```python
from build123d import *

# Parameters (mm, degrees)
SKETCH1_R           = 200
BOSS_EXTRUDE1_DEPTH = 5
CUT_EXTRUDE1_REACH  = 7
SKETCH2_R           = 5
CUT_EXTRUDE2_REACH  = 7
SKETCH3_R           = 2.75
CUT_EXTRUDE3_REACH  = 7
SKETCH4_R           = 2


with BuildPart() as part:
    # Sketch1 → Boss-Extrude1 (new body)
    with BuildSketch(Plane.XY):
        Circle(SKETCH1_R)
    extrude(amount=BOSS_EXTRUDE1_DEPTH)

    # Sketch2 → Cut-Extrude1 (cut, up to next)
    with BuildSketch(Plane.XY.offset(5), mode=Mode.PRIVATE) as cut_extrude1_sk1:
        with Locations((0, 180)):
            Circle(SKETCH2_R)
    cut_extrude1_tool1 = extrude(cut_extrude1_sk1.sketch, amount=-CUT_EXTRUDE1_REACH, mode=Mode.PRIVATE) & part.part
    add(cut_extrude1_tool1.solids().sort_by_distance((0, 180, 5))[0], mode=Mode.SUBTRACT)
    # Sketch2 → Cut-Extrude1 (cut, up to next)
    with BuildSketch(Plane.XY.offset(5), mode=Mode.PRIVATE) as cut_extrude1_sk2:
        with Locations((155.884572681, -90)):
            Circle(SKETCH2_R)
    cut_extrude1_tool2 = extrude(cut_extrude1_sk2.sketch, amount=-CUT_EXTRUDE1_REACH, mode=Mode.PRIVATE) & part.part
    add(cut_extrude1_tool2.solids().sort_by_distance((155.884573, -90, 5))[0], mode=Mode.SUBTRACT)
    # Sketch2 → Cut-Extrude1 (cut, up to next)
    with BuildSketch(Plane.XY.offset(5), mode=Mode.PRIVATE) as cut_extrude1_sk3:
        with Locations((-155.884572681, -90)):
            Circle(SKETCH2_R)
    cut_extrude1_tool3 = extrude(cut_extrude1_sk3.sketch, amount=-CUT_EXTRUDE1_REACH, mode=Mode.PRIVATE) & part.part
    add(cut_extrude1_tool3.solids().sort_by_distance((-155.884573, -90, 5))[0], mode=Mode.SUBTRACT)

    # Sketch3 → Cut-Extrude2 (cut, up to next)
    with BuildSketch(Plane.XY.offset(5), mode=Mode.PRIVATE) as cut_extrude2_sk1:
        with Locations((-60, 60)):
            Circle(SKETCH3_R)
    cut_extrude2_tool1 = extrude(cut_extrude2_sk1.sketch, amount=-CUT_EXTRUDE2_REACH, mode=Mode.PRIVATE) & part.part
    add(cut_extrude2_tool1.solids().sort_by_distance((-60, 60, 5))[0], mode=Mode.SUBTRACT)
    # Sketch3 → Cut-Extrude2 (cut, up to next)
    with BuildSketch(Plane.XY.offset(5), mode=Mode.PRIVATE) as cut_extrude2_sk2:
        with Locations((60, 60)):
            Circle(SKETCH3_R)
    cut_extrude2_tool2 = extrude(cut_extrude2_sk2.sketch, amount=-CUT_EXTRUDE2_REACH, mode=Mode.PRIVATE) & part.part
    add(cut_extrude2_tool2.solids().sort_by_distance((60, 60, 5))[0], mode=Mode.SUBTRACT)
    # Sketch3 → Cut-Extrude2 (cut, up to next)
    with BuildSketch(Plane.XY.offset(5), mode=Mode.PRIVATE) as cut_extrude2_sk3:
        with Locations((60, -60)):
            Circle(SKETCH3_R)
    cut_extrude2_tool3 = extrude(cut_extrude2_sk3.sketch, amount=-CUT_EXTRUDE2_REACH, mode=Mode.PRIVATE) & part.part
    add(cut_extrude2_tool3.solids().sort_by_distance((60, -60, 5))[0], mode=Mode.SUBTRACT)
    # Sketch3 → Cut-Extrude2 (cut, up to next)
    with BuildSketch(Plane.XY.offset(5), mode=Mode.PRIVATE) as cut_extrude2_sk4:
        with Locations((-60, -60)):
            Circle(SKETCH3_R)
    cut_extrude2_tool4 = extrude(cut_extrude2_sk4.sketch, amount=-CUT_EXTRUDE2_REACH, mode=Mode.PRIVATE) & part.part
    add(cut_extrude2_tool4.solids().sort_by_distance((-60, -60, 5))[0], mode=Mode.SUBTRACT)

    # Sketch4 → Cut-Extrude3 (cut, up to next)
    with BuildSketch(Plane.XY.offset(5), mode=Mode.PRIVATE) as cut_extrude3_sk1:
        with Locations((11, -140)):
            Circle(SKETCH4_R)
    cut_extrude3_tool1 = extrude(cut_extrude3_sk1.sketch, amount=-CUT_EXTRUDE3_REACH, mode=Mode.PRIVATE) & part.part
    add(cut_extrude3_tool1.solids().sort_by_distance((11, -140, 5))[0], mode=Mode.SUBTRACT)
    # Sketch4 → Cut-Extrude3 (cut, up to next)
    with BuildSketch(Plane.XY.offset(5), mode=Mode.PRIVATE) as cut_extrude3_sk2:
        with Locations((-11, -140)):
            Circle(SKETCH4_R)
    cut_extrude3_tool2 = extrude(cut_extrude3_sk2.sketch, amount=-CUT_EXTRUDE3_REACH, mode=Mode.PRIVATE) & part.part
    add(cut_extrude3_tool2.solids().sort_by_distance((-11, -140, 5))[0], mode=Mode.SUBTRACT)


solid = part.part
```
Work out the finished part from the listing and answer in its coordinate system (mm). Give positions to 0.01 mm unless a question says otherwise; leave off trailing zeros. Loops run counter-clockwise (first coordinate to the right, second up) from the corner with the lowest first, then second, coordinate; pieces in that order, holes last. Notation, with made-up numbers: M 64,71 L 115,71 A18 ccw 115,88 Z; hole C 53.25,-18.5 d7. An arc over 180 degrees is marked long. One line per item, written item: value. Start each with the question number.
1. Each of these flat-tipped pins is pushed along its axis until it touches: P1, Ø3, axis at y = 58, z = 0.5, coming from the -X side; P2, Ø1, axis at y = 110.5, z = 4.5, coming from the -X side; P3, Ø1, axis at x = 50, z = 4, coming from the -Y side. Where does it stop, or does it pass through?
2. Find section D-D (y = -90). Give the vertices of the cut face in (x, z).
3. Find section C-C (y = 180). Give the vertices of the cut face in (x, z), and give its area (3 significant figures).
4. Determine the mould class of faces 1 (the face through (-3, 3, 0)), 2 (the face through (190.764, 60.075, 2.465)), 3 (the face through (151.917, -93.042, 2.535)) for opening direction Y: released by +Y, released by -Y, zero draft, split by the parting line, or undercut.
5. Find the intervals of material crossed by probe 1 along Y at (x, z) = (-60, 2.3); probe 2 along X at (y, z) = (-140, 3.55); probe 3 along Y at (x, z) = (160, 3.05), in increasing order.
6. Find section B-B (z = 3.2). State how many separate pieces and enclosed holes the cut face has, and give its area (3 significant figures).
7. Find section A-A (x = 0). Give the vertices of the cut face in (y, z), and give its area (3 significant figures).
Reported:
1. P1: stops at x = -191.85
1. P2: stops at x = -167.03
1. P3: stops at y = -193.78
2. outline: M -178.61,0 L -160.88,0 L -160.88,5 L -178.61,5 Z; M -150.88,0 L 150.88,0 L 150.88,5 L -150.88,5 Z; M 160.88,0 L 178.61,0 L 178.61,5 L 160.88,5 Z
3. outline: M -87.18,0 L -5,0 L -5,5 L -87.18,5 Z; M 5,0 L 87.18,0 L 87.18,5 L 5,5 Z
3. area: 822 mm²
4. face 1: zero draft
4. face 2: split by the parting line
4. face 3: undercut
5. probe 1: y = -190.79 to -62.75, -57.25 to 57.25, 62.75 to 190.79
5. probe 2: x = -142.83 to -13, -9 to 9, 13 to 142.83
5. probe 3: y = -120 to -92.84, -87.16 to 120
6. separate pieces: 1
6. enclosed holes: 9
6. area: 125,000 mm²
7. outline: M -200,0 L 175,0 L 175,5 L -200,5 Z; M 185,0 L 200,0 L 200,5 L 185,5 Z
7. area: 1,950 mm²
